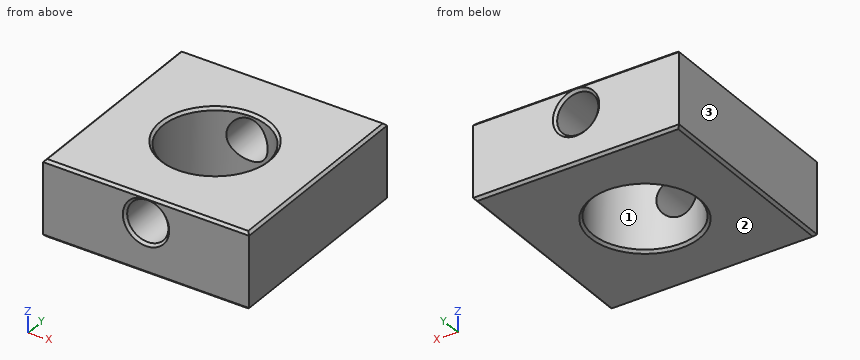
```python
from build123d import *

# Parameters (mm, degrees)
SKETCH1_W               = 20
SKETCH1_H               = 20
SKETCH1_R               = 5.05
BOSS_EXTRUDE1_DEPTH     = 7.4
CUT_EXTRUDE1_DEPTH      = 16.961202962
CUT_EXTRUDE1_DEPTH_BACK = 16.961202962
SKETCH2_R               = 2
CHAMFER1_SIZE           = 0.25


with BuildPart() as part:
    # Sketch1 → Boss-Extrude1 (new body)
    with BuildSketch(Plane.XY):
        Rectangle(SKETCH1_W, SKETCH1_H)
        Circle(SKETCH1_R, mode=Mode.SUBTRACT)
    extrude(amount=BOSS_EXTRUDE1_DEPTH)

    # Sketch2 → Cut-Extrude1 (cut, two sides: drawn at the far end of the back side and taken through both)
    with BuildSketch(Plane(origin=(0, 0, 0), x_dir=(1, 0, 0), z_dir=(0, 1, 0)).offset(-CUT_EXTRUDE1_DEPTH_BACK)):
        with Locations(Location((0, -4.9, 0), (0, 0, 270))):
            Circle(SKETCH2_R)
    extrude(amount=CUT_EXTRUDE1_DEPTH + CUT_EXTRUDE1_DEPTH_BACK, mode=Mode.SUBTRACT)

    # Chamfer1
    chamfer1_edges = [part.edges().sort_by_distance(p)[0] for p in [
        (-5.05, 0, 0),
        (-5.05, 0, 7.4),
        (-10, 0, 7.4),
        (0, -10, 7.4),
        (0, -10, 2.9),
        (0, 10, 2.9),
        (10, 0, 7.4),
        (0, -10, 0),
        (-10, 0, 0),
        (0, 10, 0),
        (10, 0, 0),
        (0, 10, 7.4),
    ]]
    chamfer(chamfer1_edges, length=CHAMFER1_SIZE - 0.0001)  # a hair under: the kernel refuses the full size


solid = part.part
```
Check sheet for the modelled part. Datum: model origin and axes. Units: mm. Face numbers are marked on the shaded views. Coordinates: 2 decimals unless noted, no trailing zeros. Loops run counter-clockwise (first coordinate to the right, second up) from the corner with the lowest first, then second, coordinate; pieces in that order, holes last.
1) Sectioned sample at C-C (x = 0). Count the separate pieces of the cut face and the enclosed holes in it, and give its area (3 significant figures).
2) Sectioned sample at A-A (z = 4.9). Record the boundary of the cut face in (x, y), and give its area (3 significant figures).
3) Release check for a two-part mould opening along X. For the marked faces 1, 2 and 3 record: released by +X, released by -X, zero draft, split by the parting line, or undercut.
4) Sectioned sample at B-B (y = 0). Record the boundary of the cut face in (x, z).
5) Material ranges on probe 1 along Z at (x, y) = (0, 6.3); probe 2 along X at (y, z) = (-6.2, 4.9); probe 3 along Y at (x, z) = (-0.5, 1.75), recorded low to high.
6) Sectioned sample at D-D (z = 2). Record the boundary of the cut face in (x, y), and give its area (3 significant figures).
Check sheet entries:
1. separate pieces: 4
1. enclosed holes: 0
1. area: 33.3 mm2
2. outline: (-10, -10) - (-2.25, -10) - (-2, -9.75) - (-2, -4.64) arc R5.05 cw to (-2, 4.64) - (-2, 9.75) - (-2.25, 10) - (-10, 10) - close; (2, -9.75) - (2.25, -10) - (10, -10) - (10, 10) - (2.25, 10) - (2, 9.75) - (2, 4.64) arc R5.05 cw to (2, -4.64) - close
2. area: 279 mm2
3. face 1: undercut
3. face 2: zero draft
3. face 3: released by -X
4. outline: (-10, 0.25) - (-9.75, 0) - (-5.3, 0) - (-5.05, 0.25) - (-5.05, 7.15) - (-5.3, 7.4) - (-9.75, 7.4) - (-10, 7.15) - close; (5.05, 0.25) - (5.3, 0) - (9.75, 0) - (10, 0.25) - (10, 7.15) - (9.75, 7.4) - (5.3, 7.4) - (5.05, 7.15) - close
5. probe 1: z = 0 to 2.9, 6.9 to 7.4
5. probe 2: x = -10 to -2, 2 to 10
5. probe 3: y = -10 to -5.03, 5.03 to 10
6. outline: (-10, -10) - (10, -10) - (10, 10) - (-10, 10) - close; hole circle Ø10.1 at (0, 0)
6. area: 320 mm2
